from build123d import *

# Parameters (mm, degrees)
SKETCH1_W           = 65
SKETCH1_H           = 5
BOSS_EXTRUDE1_DEPTH = 8
SKETCH2_R           = 1.75
CUT_EXTRUDE1_DEPTH  = 37.504037204
FILLET1_R           = 2


with BuildPart() as part:
    # Sketch1 → Boss-Extrude1 (new body)
    with BuildSketch(Plane.XY):
        with Locations((2.763929619, 0)):
            Rectangle(SKETCH1_W, SKETCH1_H)
    extrude(amount=-BOSS_EXTRUDE1_DEPTH)

    # Sketch2 → Cut-Extrude1 (cut, through all)
    with BuildSketch(Plane(origin=(0, 2.5, 0), x_dir=(1, 0, 0), z_dir=(0, 1, 0))):
        with Locations(Location((32.763929619, 4, 0), (0, 0, 180))):
            Circle(SKETCH2_R)
        with Locations((-27.236070381, 4)):
            Circle(SKETCH2_R)
    extrude(amount=-CUT_EXTRUDE1_DEPTH, mode=Mode.SUBTRACT)

    # Fillet1
    # the kernel refuses this fillet: 2 mm, written as the material it takes off along each edge
    with BuildSketch(Plane(origin=(33.263929619, 0.5, -6), x_dir=(0, 0, -1), z_dir=(0, 1, 0))) as fillet1_piece_1_section:
        Polygon((0, 0), (FILLET1_R, 0), (FILLET1_R, -FILLET1_R), (0, -FILLET1_R), align=None)
    fillet1_piece_1 = extrude(amount=FILLET1_R, mode=Mode.PRIVATE)
    fillet1_piece_1 = fillet1_piece_1 - Plane(origin=(33.263929619, 0.5, -6), x_dir=(-0.7071067811865475, 0, 0.7071067811865475), z_dir=(0, 1, 0)) * Sphere(FILLET1_R, mode=Mode.PRIVATE)
    add(fillet1_piece_1, mode=Mode.SUBTRACT)
    with BuildSketch(Plane(origin=(33.263929619, -0.5, -6), x_dir=(1, 0, 0), z_dir=(0, 0, -1))) as fillet1_piece_2_section:
        Polygon((0, 0), (FILLET1_R, 0), (FILLET1_R, FILLET1_R), (0, FILLET1_R), align=None)
    fillet1_piece_2 = extrude(amount=FILLET1_R, mode=Mode.PRIVATE)
    fillet1_piece_2 = fillet1_piece_2 - Plane(origin=(33.263929619, -0.5, -6), x_dir=(-0.7071067811865475, 0.7071067811865475, 0), z_dir=(0, 0, -1)) * Sphere(FILLET1_R, mode=Mode.PRIVATE)
    add(fillet1_piece_2, mode=Mode.SUBTRACT)
    with BuildSketch(Plane(origin=(-27.736070381, 0.5, -6), x_dir=(-1, 0, 0), z_dir=(0, 1, 0))) as fillet1_piece_3_section:
        Polygon((0, 0), (FILLET1_R, 0), (FILLET1_R, -FILLET1_R), (0, -FILLET1_R), align=None)
    fillet1_piece_3 = extrude(amount=FILLET1_R, mode=Mode.PRIVATE)
    fillet1_piece_3 = fillet1_piece_3 - Plane(origin=(-27.736070381, 0.5, -6), x_dir=(0.7071067811865475, 0, 0.7071067811865475), z_dir=(0, 1, 0)) * Sphere(FILLET1_R, mode=Mode.PRIVATE)
    add(fillet1_piece_3, mode=Mode.SUBTRACT)
    with BuildSketch(Plane(origin=(-27.736070381, -0.5, -6), x_dir=(0, 0, -1), z_dir=(-1, 0, 0))) as fillet1_piece_4_section:
        Polygon((0, 0), (FILLET1_R, 0), (FILLET1_R, FILLET1_R), (0, FILLET1_R), align=None)
    fillet1_piece_4 = extrude(amount=FILLET1_R, mode=Mode.PRIVATE)
    fillet1_piece_4 = fillet1_piece_4 - Plane(origin=(-27.736070381, -0.5, -6), x_dir=(0, 0.7071067811865475, 0.7071067811865475), z_dir=(-1, 0, 0)) * Sphere(FILLET1_R, mode=Mode.PRIVATE)
    add(fillet1_piece_4, mode=Mode.SUBTRACT)
    with BuildSketch(Plane(origin=(-27.736070381, 0.5, -2), x_dir=(-1, 0, 0), z_dir=(0, 1, 0))) as fillet1_piece_5_section:
        Polygon((0, 0), (FILLET1_R, 0), (FILLET1_R, FILLET1_R), (0, FILLET1_R), align=None)
    fillet1_piece_5 = extrude(amount=FILLET1_R, mode=Mode.PRIVATE)
    fillet1_piece_5 = fillet1_piece_5 - Plane(origin=(-27.736070381, 0.5, -2), x_dir=(0.7071067811865475, 0, -0.7071067811865475), z_dir=(0, 1, 0)) * Sphere(FILLET1_R, mode=Mode.PRIVATE)
    add(fillet1_piece_5, mode=Mode.SUBTRACT)
    with BuildSketch(Plane(origin=(33.263929619, 0.5, -2), x_dir=(0, 0, 1), z_dir=(0, 1, 0))) as fillet1_piece_6_section:
        Polygon((0, 0), (FILLET1_R, 0), (FILLET1_R, FILLET1_R), (0, FILLET1_R), align=None)
    fillet1_piece_6 = extrude(amount=FILLET1_R, mode=Mode.PRIVATE)
    fillet1_piece_6 = fillet1_piece_6 - Plane(origin=(33.263929619, 0.5, -2), x_dir=(-0.7071067811865475, 0, -0.7071067811865475), z_dir=(0, 1, 0)) * Sphere(FILLET1_R, mode=Mode.PRIVATE)
    add(fillet1_piece_6, mode=Mode.SUBTRACT)
    with BuildSketch(Plane(origin=(33.263929619, -0.5, -2), x_dir=(1, 0, 0), z_dir=(0, 0, 1))) as fillet1_piece_7_section:
        Polygon((0, 0), (FILLET1_R, 0), (FILLET1_R, -FILLET1_R), (0, -FILLET1_R), align=None)
    fillet1_piece_7 = extrude(amount=FILLET1_R, mode=Mode.PRIVATE)
    fillet1_piece_7 = fillet1_piece_7 - Plane(origin=(33.263929619, -0.5, -2), x_dir=(-0.7071067811865475, 0.7071067811865475, 0), z_dir=(0, 0, 1)) * Sphere(FILLET1_R, mode=Mode.PRIVATE)
    add(fillet1_piece_7, mode=Mode.SUBTRACT)
    with BuildSketch(Plane(origin=(-27.736070381, -0.5, -2), x_dir=(0, 0, 1), z_dir=(-1, 0, 0))) as fillet1_piece_8_section:
        Polygon((0, 0), (FILLET1_R, 0), (FILLET1_R, -FILLET1_R), (0, -FILLET1_R), align=None)
    fillet1_piece_8 = extrude(amount=FILLET1_R, mode=Mode.PRIVATE)
    fillet1_piece_8 = fillet1_piece_8 - Plane(origin=(-27.736070381, -0.5, -2), x_dir=(0, 0.7071067811865475, -0.7071067811865475), z_dir=(-1, 0, 0)) * Sphere(FILLET1_R, mode=Mode.PRIVATE)
    add(fillet1_piece_8, mode=Mode.SUBTRACT)
    with BuildSketch(Plane(origin=(35.263929619, 0.5, -8), x_dir=(-1, 0, 0), z_dir=(0, -1, 0)), Plane(origin=(-29.736070381, -0.5, 0), x_dir=(0, 0, -1), z_dir=(0, 1, 0))) as fillet1_piece_9:
        with BuildLine():
            CenterArc((FILLET1_R, -FILLET1_R), FILLET1_R, 90, 90)
            Line((0, -FILLET1_R), (0, 0))
            Line((0, 0), (FILLET1_R, 0))
        make_face()
    extrude(amount=1, mode=Mode.SUBTRACT)
    with BuildSketch(Plane(origin=(-27.736070381, 2.5, -8), x_dir=(0, 0, 1), z_dir=(1, 0, 0)), Plane(origin=(33.263929619, -2.5, 0), x_dir=(0, 1, 0), z_dir=(-1, 0, 0))) as fillet1_piece_10:
        with BuildLine():
            CenterArc((FILLET1_R, FILLET1_R), FILLET1_R, 180, 90)
            Line((0, FILLET1_R), (0, 0))
            Line((0, 0), (FILLET1_R, 0))
        make_face()
    extrude(amount=61, mode=Mode.SUBTRACT)
    with BuildSketch(Plane(origin=(-27.236070381, 2.5, -4), x_dir=(1, 0, 0), z_dir=(0, 0, 1))) as fillet1_piece_11:
        with BuildLine():
            CenterArc((1.75 + FILLET1_R, -FILLET1_R), FILLET1_R, 90, 90)
            Line((1.75, -FILLET1_R), (1.75, 0))
            Line((1.75, 0), (1.75 + FILLET1_R, 0))
        make_face()
    revolve(axis=Axis((-27.236070381, 2.5, -4), (0, 1, 0)), mode=Mode.SUBTRACT)
    with BuildSketch(Plane(origin=(-27.236070381, -2.5, -4), x_dir=(1, 0, 0), z_dir=(0, 0, 1))) as fillet1_piece_12:
        with BuildLine():
            CenterArc((1.75 + FILLET1_R, FILLET1_R), FILLET1_R, 180, 90)
            Line((1.75 + FILLET1_R, 0), (1.75, 0))
            Line((1.75, 0), (1.75, FILLET1_R))
        make_face()
    revolve(axis=Axis((-27.236070381, -2.5, -4), (0, 1, 0)), mode=Mode.SUBTRACT)
    with BuildSketch(Plane(origin=(32.763929619, -2.5, -4), x_dir=(-1, 0, 0), z_dir=(0, 0, -1))) as fillet1_piece_13:
        with BuildLine():
            CenterArc((1.75 + FILLET1_R, FILLET1_R), FILLET1_R, 180, 90)
            Line((1.75 + FILLET1_R, 0), (1.75, 0))
            Line((1.75, 0), (1.75, FILLET1_R))
        make_face()
    revolve(axis=Axis((32.763929619, -2.5, -4), (0, 1, 0)), mode=Mode.SUBTRACT)
    with BuildSketch(Plane(origin=(32.763929619, 2.5, -4), x_dir=(-1, 0, 0), z_dir=(0, 0, -1))) as fillet1_piece_14:
        with BuildLine():
            CenterArc((1.75 + FILLET1_R, -FILLET1_R), FILLET1_R, 90, 90)
            Line((1.75, -FILLET1_R), (1.75, 0))
            Line((1.75, 0), (1.75 + FILLET1_R, 0))
        make_face()
    revolve(axis=Axis((32.763929619, 2.5, -4), (0, 1, 0)), mode=Mode.SUBTRACT)
    with BuildSketch(Plane(origin=(-29.736070381, -0.5, -8), x_dir=(0, 0, 1), z_dir=(0, 1, 0)), Plane(origin=(35.263929619, 0.5, 0), x_dir=(-1, 0, 0), z_dir=(0, -1, 0))) as fillet1_piece_15:
        with BuildLine():
            CenterArc((FILLET1_R, FILLET1_R), FILLET1_R, 180, 90)
            Line((0, FILLET1_R), (0, 0))
            Line((0, 0), (FILLET1_R, 0))
        make_face()
    extrude(amount=1, mode=Mode.SUBTRACT)
    with BuildSketch(Plane(origin=(-27.736070381, 2.5, 0), x_dir=(0, 0, -1), z_dir=(1, 0, 0)), Plane(origin=(33.263929619, -2.5, -8), x_dir=(0, 1, 0), z_dir=(-1, 0, 0))) as fillet1_piece_16:
        with BuildLine():
            CenterArc((FILLET1_R, -FILLET1_R), FILLET1_R, 90, 90)
            Line((0, -FILLET1_R), (0, 0))
            Line((0, 0), (FILLET1_R, 0))
        make_face()
    extrude(amount=61, mode=Mode.SUBTRACT)
    with BuildSketch(Plane(origin=(-29.736070381, 2.5, -2), x_dir=(1, 0, 0), z_dir=(0, 0, -1)), Plane(origin=(-29.736070381, -2.5, -2), x_dir=(0, 1, 0), z_dir=(0, 0, -1))) as fillet1_piece_17:
        with BuildLine():
            CenterArc((FILLET1_R, FILLET1_R), FILLET1_R, 180, 90)
            Line((0, FILLET1_R), (0, 0))
            Line((0, 0), (FILLET1_R, 0))
        make_face()
    extrude(amount=4, mode=Mode.SUBTRACT)
    with BuildSketch(Plane(origin=(35.263929619, 2.5, -2), x_dir=(-1, 0, 0), z_dir=(0, 0, -1)), Plane(origin=(35.263929619, -2.5, -2), x_dir=(0, 1, 0), z_dir=(0, 0, -1))) as fillet1_piece_18:
        with BuildLine():
            CenterArc((FILLET1_R, -FILLET1_R), FILLET1_R, 90, 90)
            Line((0, -FILLET1_R), (0, 0))
            Line((0, 0), (FILLET1_R, 0))
        make_face()
    extrude(amount=4, mode=Mode.SUBTRACT)


solid = part.part
Work out the finished part from the listing and answer in its coordinate system (mm). Round coordinates to 2 decimals unless told otherwise and drop trailing zeros. Loops run counter-clockwise (first coordinate to the right, second up) from the corner with the lowest first, then second, coordinate; pieces in that order, holes last. Notation, with made-up numbers: (17.5, 53) - (62.5, 53) arc R11 ccw to (62.5, 64) - close; hole circle Ø4 at (66, 71). An arc over 180 degrees is marked (long way). One line per item, written item: value.
Q1. Find section B-B on x = 4.5. Give the vertices of the cut face in (y, z).
Check values:
outline: (-2.5, -6) arc R2 ccw to (-0.5, -8) - (0.5, -8) arc R2 ccw to (2.5, -6) - (2.5, -2) arc R2 ccw to (0.5, 0) - (-0.5, 0) arc R2 ccw to (-2.5, -2) - close
Q2. Find section C-C on z = -4. Give the vertices of the cut face in (x, y), and give its area (3 significant figures).
Check values:
outline: (-29.74, -0.5) arc R2 ccw to (-29.36, -1.67) arc R2 ccw to (-28.99, -0.5) - (-28.99, 0.5) arc R2 ccw to (-29.36, 1.67) arc R2 ccw to (-29.74, 0.5) - close; (-25.49, -0.5) arc R2 ccw to (-23.49, -2.5) - (29.01, -2.5) arc R2 ccw to (31.01, -0.5) - (31.01, 0.5) arc R2 ccw to (29.01, 2.5) - (-23.49, 2.5) arc R2 ccw to (-25.49, 0.5) - close; (34.51, -0.5) arc R2 ccw to (34.89, -1.67) arc R2 ccw to (35.26, -0.5) - (35.26, 0.5) arc R2 ccw to (34.89, 1.67) arc R2 ccw to (34.51, 0.5) - close
area: 283 mm2
Q3. Find section A-A on y = 1.25. Give the vertices of the cut face in (x, z).
Check values:
outline: (-29.59, -6) arc R1.85 ccw to (-27.74, -7.85) - (33.26, -7.85) arc R1.85 ccw to (35.12, -6) - (35.12, -2) arc R1.85 ccw to (33.26, -0.15) - (-27.74, -0.15) arc R1.85 ccw to (-29.59, -2) - close; hole circle Ø3.79 at (-27.24, -4); hole circle Ø3.79 at (32.76, -4)
Q4. Straight lines are drawn through the part: probe 1 along X at (y, z) = (1.85, -2); probe 2 along X at (y, z) = (1.4, -4.75); probe 3 along Z at (x, y) = (33.5, 0.55). For each, find the intervals that lie inside material, in ascending order.
Check values:
probe 1: -29.21 to -28.32, -26.15 to 31.68, 33.85 to 34.74
probe 2: -29.52 to -29.05, -25.42 to 30.95, 34.58 to 35.05
probe 3: -7.99 to -5.59, -2.41 to -0.01
Q5. The mould has two halves that part along X. Classify faces 1 (the cylindrical face through (-28.984, 0.007, -4.077)), 2 (the cylindrical face through (3.19, -1.93, -0.6)), 3 (the cylindrical face through (-29.135, -0.007, -7.43)): +X half, -X half, draft (parallel to the pull), parting line (faces both ways), or undercut.
Check values:
face 1: undercut
face 2: draft
face 3: -X half
Q6. This flat-tipped pin is pushed along its axis until it touches: pin 1 Ø2 at (x, z) = (-27.24, -4) entering from -Y. Where does it stop, or does it pass through?
Check values:
pin 1: through
